Autodesk Inventor part; units mm, degrees
ref_plane "YZ Plane" through (0, 0, 0) normal (1, 0, 0) x (0, 1, 0)
ref_plane "XZ Plane" through (0, 0, 0) normal (0, 1, 0) x (-1, 0, 0)
ref_plane "XY Plane" through (0, 0, 0) normal (0, 0, 1) x (1, 0, 0)
sketch "Sketch1" plane through (0, 0, 0) normal (0, 0, 1) x (1, 0, 0)
  arc A0 (0, -144.3376) -> (125, 72.1688) centre (-125, 72.1688) ccw
  arc A1 (-125, 72.1688) -> (0, -144.3376) centre (125, 72.1688) ccw
  arc A2 (125, 72.1688) -> (-125, 72.1688) centre (0, -144.3376) ccw
  line L0 (-125, 72.1688) -> (0, 0) construction
  line L1 (0, 0) -> (125, 72.1688) construction
  line L2 (0, 0) -> (0, -144.3376) construction
  circle A3 centre (0, 0) radius 100
  arc A4 (-131.25, 82.9941) -> (-137.5, 72.1688) centre (-125, 72.1688) ccw
  arc A5 (137.5, 72.1688) -> (131.25, 82.9941) centre (125, 72.1688) ccw
  arc A6 (-6.25, -155.1629) -> (6.25, -155.1629) centre (0, -144.3376) ccw
  arc A7 (-137.5, 72.1688) -> (-6.25, -155.1629) centre (125, 72.1688) ccw
  arc A8 (131.25, 82.9941) -> (-131.25, 82.9941) centre (0, -144.3376) ccw
  arc A9 (6.25, -155.1629) -> (137.5, 72.1688) centre (-125, 72.1688) ccw
  line L3 (-100, 100) -> (100, 100)
  line L4 (100, 100) -> (100, -100)
  line L5 (100, -100) -> (-100, -100)
  line L6 (-100, -100) -> (-100, 100)
  point P0 (0, 0)
  point P1 (0, 0)
  dimension "d0" = 200
  dimension "d2" = 250
  dimension "d3" = 12.5
extrude "Extrusion1" add sketch "Sketch1" along normal blind 12.5 contours A1 L5 A0 | A0 L5 A9 A6 A7 A1 | L5 A3 L4 A0 | A0 L4 A9 L5 | L5 A7 L6 A1 | A1 L6 A3 L5 | L4 A2 A0 | A0 A2 L4 A8 A5 A9 | A3 | L6 A7 A4 A8 A2 A1 | A1 A2 L6 | A3 L3 A2 L4 | L6 A2 L3 A3 | A2 L3 A8 L4 | L3 A2 | L6 A8 L3 A2 | A2 L3 A8
sketch "Sketch2" plane through (0, 0, 12.5) normal (0, 0, 1) x (1, 0, 0)
  arc A0 (131.25, 82.9941) -> (-131.25, 82.9941) centre (0, -144.3376) ccw
  arc A1 (-131.25, 82.9941) -> (-137.5, 72.1688) centre (-125, 72.1688) ccw
  arc A2 (-137.5, 72.1688) -> (-6.25, -155.1629) centre (125, 72.1688) ccw
  circle A3 centre (-125, 72.1688) radius 4.05
  circle A4 centre (125, 72.1688) radius 4.05
  circle A5 centre (0, -144.3376) radius 4.05
  point P0 (0, 0)
  dimension "d6" = 8.1
extrude "Extrusion2" cut sketch "Sketch2" against normal through all
sketch "Sketch3" plane through (0, 0, 12.5) normal (0, 0, 1) x (1, 0, 0)
  circle A0 centre (0, 0) radius 100.05
  dimension "d10" = 200.1
extrude "Extrusion3" cut sketch "Sketch3" against normal blind 1.5
sketch "Sketch5" plane through (0, 0, 12.5) normal (0, 0, 1) x (1, 0, 0)
  circle A0 centre (125, 72.1688) radius 4.05
  circle A1 centre (-125, 72.1688) radius 4.05
  circle A2 centre (0, -144.3376) radius 4.05
hole "Hole1" at (0, -144.3376, 12.5) at (-125, 72.1688, 12.5) at (125, 72.1688, 12.5) direction (0, 0, -1) diameter 8.1 end through all
sketch "Sketch7" plane through (0, 0, 11) normal (0, 0, 1) x (1, 0, 0)
  circle A0 centre (0, 0) radius 100.05
  arc A1 (-36.8356, 93.0223) -> (36.8356, 93.0223) centre (0, 100.05) ccw
  dimension "d30" = 37.5
extrude "Extrusion5" cut sketch "Sketch7" against normal blind 2 contours A1 A0 picked at (-7.0348, 87.6172)
sketch "Sketch9" plane through (0, 0, 9) normal (0, 0, 1) x (1, 0, 0)
  arc A0 (-36.8356, 93.0223) -> (36.8356, 93.0223) centre (0, 100.05) ccw
  circle A1 centre (0, 100.05) radius 12.5
  dimension "d39" = 25
extrude "Extrusion7" cut sketch "Sketch9" along normal through all both and the other way through all
properties part number "build plate"
Geometry check sheet. Reference: the model listing, model coordinates, mm. A direction names the side the tool comes from. Round coordinates to 2 decimals unless told otherwise and drop trailing zeros. Write each loop counter-clockwise with the first axis right and the second up, starting at its lowest first coordinate (ties: lowest second). Pieces come first, ordered by that corner, then holes. Notation, with made-up numbers: (76, 53) -> (85, 53) arc R21 cw to (85, 72) -> close; hole circle Ø7 at (-32, 30.25). An arc over 180 degrees is marked (long way). Put each result on its own line as item: value.
1) Cross-section at B-B, the plane x = 125. Enter the section's corners in (y, z), plus the area to 3 significant figures.
Recorded:
outline: (-7.87, 0) -> (68.12, 0) -> (68.12, 12.5) -> (-7.87, 12.5) -> close; (76.22, 0) -> (86.49, 0) -> (86.49, 12.5) -> (76.22, 12.5) -> close
area: 1,080 mm2
2) Cross-section at A-A, the plane x = 0. Enter the section's corners in (y, z).
Recorded:
outline: (-156.84, 0) -> (-148.39, 0) -> (-148.39, 12.5) -> (-156.84, 12.5) -> close; (-140.29, 0) -> (87.55, 0) -> (87.55, 9) -> (62.55, 9) -> (62.55, 11) -> (-100.05, 11) -> (-100.05, 12.5) -> (-140.29, 12.5) -> close; (112.55, 0) -> (118.16, 0) -> (118.16, 12.5) -> (112.55, 12.5) -> close
3) Cross-section at D-D, the plane x = -95. Enter the section's corners in (y, z), plus the area to 3 significant figures.
Recorded:
outline: (-71.03, 0) -> (100.37, 0) -> (100.37, 12.5) -> (31.38, 12.5) -> (31.38, 11) -> (-31.38, 11) -> (-31.38, 12.5) -> (-71.03, 12.5) -> close
area: 2,050 mm2
4) Thickness scan on probe 1 along Y at (x, z) = (0, 6.5); probe 2 along Y at (x, z) = (0, 9.9); probe 3 along Z at (x, y) = (-29, 1). Record the ranges inside material, lowest first. Write a range as from..to.
Recorded:
probe 1: y = -156.84..-148.39, -140.29..87.55, 112.55..118.16
probe 2: y = -156.84..-148.39, -140.29..62.55, 112.55..118.16
probe 3: z = 0..11
5) Depth check by flat-ended pin: P1, Ø1, axis at x = -96, z = 10, coming from the -Y side; P2, Ø4, axis at y = -119.5, z = 10, coming from the -X side; P3, Ø1.5, axis at x = -85.5, z = 6, coming from the +Y side. Enter the tip coordinate at first touch or a pass-through.
Recorded:
P1: stops at y = -70.26
P2: stops at x = -56.47
P3: stops at y = 104.1
6) Cross-section at C-C, the plane z = 5. Enter the section's corners in (x, y), plus the area to 3 significant figures.
Recorded:
outline: (-137.5, 72.17) arc R262.5 ccw to (-6.25, -155.16) arc R12.5 ccw to (6.25, -155.16) arc R262.5 ccw to (137.5, 72.17) arc R12.5 ccw to (131.25, 82.99) arc R262.5 ccw to (-131.25, 82.99) arc R12.5 ccw to start; hole circle Ø8.1 at (-125, 72.17); hole circle Ø25 at (0, 100.05); hole circle Ø8.1 at (0, -144.34); hole circle Ø8.1 at (125, 72.17)
area: 53,700 mm2
7) Access from +Z, -Z, +X, -X, +Y, -Y to the whole of each face (thin tool, end or side, straight path). Record for faces 5 (the face through (-101.363, -60.744, 6.162)), 6 (the face through (-0.726, 62.557, 10.014)).
Recorded:
face 5: +Z, -Z, -X, -Y
face 6: +Z
8) Release check for a two-part mould opening along Y. For faces 1 (the face through (128.86, 73.39, 6.34)), 2 (the face through (-1, -2, 11)), 3 (the face through (103.29, -57.41, 6.16)), 4 (the face through (71, 73, 12.5)) record: pulls with the +Y half, pulls with the -Y half, needs draft (parallel to the pull), parting line crosses it, or undercut.
Recorded:
face 1: undercut
face 2: undercut
face 3: pulls with the -Y half
face 4: needs draft
